CAD build for the part. Positions are in the model's coordinates, mm. Coordinates: 2 decimals unless noted, no trailing zeros. Loops run counter-clockwise (first coordinate to the right, second up) from the corner with the lowest first, then second, coordinate; pieces in that order, holes last. Notation, with made-up numbers: (61.5, 53.5) -> (94.5, 53.5) arc R27 cw to (94.5, 70.5) -> close; hole circle Ø3 at (87, 31.25). An arc over 180 degrees is marked (long way). Answer as a JSON object with one key per item and string values. Group by question number.
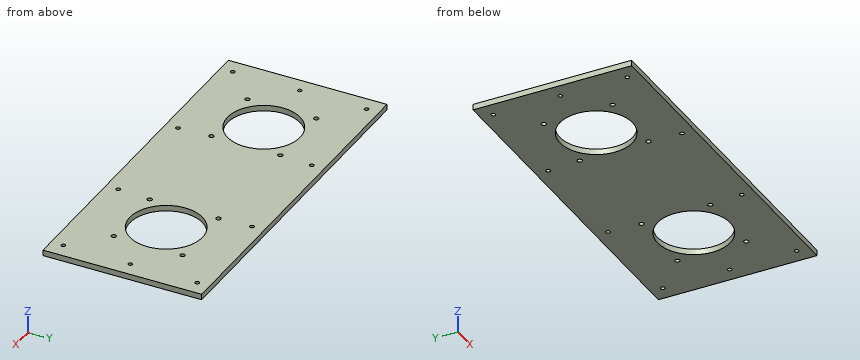
from build123d import *

# Parameters (mm, degrees)
ESQUISSE1_W             = 372
ESQUISSE1_H             = 166
ESQUISSE1_R             = 2.2
BOSS_EXTRU_1_DEPTH      = 6
ESQUISSE2_R             = 38
ESQUISSE2_R_2           = 2.5
ENL_V_MAT_EXTRU_1_DEPTH = 7


with BuildPart() as part:
    # Esquisse1 → Boss.-Extru.1 (new body)
    with BuildSketch(Plane.XY):
        Rectangle(ESQUISSE1_W, ESQUISSE1_H)
        with Locations((-170, 70)):
            Circle(ESQUISSE1_R, mode=Mode.SUBTRACT)
        with Locations((-60, 70)):
            Circle(ESQUISSE1_R, mode=Mode.SUBTRACT)
        with Locations((60, 70)):
            Circle(ESQUISSE1_R, mode=Mode.SUBTRACT)
        with Locations((170, 70)):
            Circle(ESQUISSE1_R, mode=Mode.SUBTRACT)
        with Locations((170, -70)):
            Circle(ESQUISSE1_R, mode=Mode.SUBTRACT)
        with Locations((60, -70)):
            Circle(ESQUISSE1_R, mode=Mode.SUBTRACT)
        with Locations((-60, -70)):
            Circle(ESQUISSE1_R, mode=Mode.SUBTRACT)
        with Locations((-170, -70)):
            Circle(ESQUISSE1_R, mode=Mode.SUBTRACT)
        with Locations((-170, 0)):
            Circle(ESQUISSE1_R, mode=Mode.SUBTRACT)
        with Locations((170, 0)):
            Circle(ESQUISSE1_R, mode=Mode.SUBTRACT)
    extrude(amount=BOSS_EXTRU_1_DEPTH)

    # Esquisse2 → Enlèv. mat.-Extru.1 (cut, through all)
    with BuildSketch(Plane.XY.offset(6)):
        with Locations((-98, 0)):
            Circle(ESQUISSE2_R)
        with Locations((-134, 36)):
            Circle(ESQUISSE2_R_2)
        with Locations((-134, -36)):
            Circle(ESQUISSE2_R_2)
        with Locations((-62, -36)):
            Circle(ESQUISSE2_R_2)
        with Locations((-62, 36)):
            Circle(ESQUISSE2_R_2)
        with Locations((62, 36)):
            Circle(ESQUISSE2_R_2)
        with Locations((62, -36)):
            Circle(ESQUISSE2_R_2)
        with Locations((134, -36)):
            Circle(ESQUISSE2_R_2)
        with Locations((134, 36)):
            Circle(ESQUISSE2_R_2)
        with Locations((98, 0)):
            Circle(ESQUISSE2_R)
    extrude(amount=-ENL_V_MAT_EXTRU_1_DEPTH, mode=Mode.SUBTRACT)


solid = part.part
Item 1: Band-saw the part on B-B, the plane y = -7. List the corners of the cut face in (x, z), and give its area (3 significant figures).
Item 2: Band-saw the part on C-C, the plane y = 19.5. List the corners of the cut face in (x, z).
Item 3: Drill centre lines: L1, parallel to Y at x = 170, z = 4.2; L2, parallel to X at y = -7, z = 0.8; L3, parallel to X at y = -27, z = 2.5. Where is each one in solid material? Low to high.
Item 4: Band-saw the part on A-A, the plane z = 1.4. Count the separate pieces of the cut face and the enclosed holes in it, and give its area (3 significant figures).
Reply:
{
 "1": {"outline": "(-186, 0) -> (-135.35, 0) -> (-135.35, 6) -> (-186, 6) -> close; (-60.65, 0) -> (60.65, 0) -> (60.65, 6) -> (-60.65, 6) -> close; (135.35, 0) -> (186, 0) -> (186, 6) -> (135.35, 6) -> close", "area": "1,340 mm²"},
 "2": {"outline": "(-186, 0) -> (-130.62, 0) -> (-130.62, 6) -> (-186, 6) -> close; (-65.38, 0) -> (65.38, 0) -> (65.38, 6) -> (-65.38, 6) -> close; (130.62, 0) -> (186, 0) -> (186, 6) -> (130.62, 6) -> close"},
 "3": {"L1": "-83 to -72.2, -67.8 to -2.2, 2.2 to 67.8, 72.2 to 83", "L2": "-186 to -135.35, -60.65 to 60.65, 135.35 to 186", "L3": "-186 to -124.74, -71.26 to 71.26, 124.74 to 186"},
 "4": {"separate pieces": "1", "enclosed holes": "20", "area": "52,400 mm²"}
}
